Read the model definition and answer for the solid it produces. Units are mm, in the model's axes. Coordinates: 2 decimals unless noted, no trailing zeros. Loops run counter-clockwise (first coordinate to the right, second up) from the corner with the lowest first, then second, coordinate; pieces in that order, holes last. Notation, with made-up numbers: M -29,37 L 10,37 A8 cw 10,50 Z; hole C 6.5,46.5 d11. An arc over 180 degrees is marked long. Put each result on its own line as item: value.
from build123d import *

# Parameters (mm, degrees)
BOSS_EXTRUDE2_REACH      = 243.079
BOSS_EXTRUDE2_END_RADIUS = 266.319
SKETCH10_R               = 25.4
SKETCH11_R               = 12.7
CUT_EXTRUDE1_DEPTH       = 190.754
CIRPATTERN1_COUNT        = 6


with BuildPart() as part:
    # Sketch1 → Revolve1 (revolve)
    with BuildSketch(Plane(origin=(0, 0, 0), x_dir=(1, 0, 0), z_dir=(0, 1, 0)), mode=Mode.PRIVATE) as revolve1_sk:
        with BuildLine():
            Line((-148.59, 0), (-140.97, 0))
            Line((-140.97, 0), (-140.97, 12.391039743))
            ThreePointArc((-140.97, 12.391039743), (-134.615921102, 34.866271953), (-117.434796957, 50.687755913))
            ThreePointArc((-117.434796957, 50.687755913), (-60.367509579, 71.617582047), (0, 78.72368491))
            Line((0, 78.72368491), (0, 85.07368491))
            ThreePointArc((0, 85.07368491), (-61.842045719, 77.794008454), (-120.303258046, 56.352950612))
            ThreePointArc((-120.303258046, 56.352950612), (-131.462846302, 48.602983737), (-140.081763243, 38.1))
            Line((-140.081763243, 38.1), (-149.225, 38.1))
            Line((-149.225, 38.1), (-149.225, 25.4))
            Line((-149.225, 25.4), (-152.4, 25.4))
            Line((-152.4, 25.4), (-156.21, 13.674025723))
            Line((-156.21, 13.674025723), (-156.21, 9.503030405))
            Line((-156.21, 9.503030405), (-152.4, 12.7))
            Line((-152.4, 12.7), (-148.59, 12.7))
            Line((-148.59, 12.7), (-148.59, 0))
        make_face()
    revolve(revolve1_sk.sketch.rotate(Axis((0, 0, -78.72368491), (0, 0, -1)), 180), axis=Axis((0, 0, -78.72368491), (0, 0, -1)))

    # Boss-Extrude2: up to this sphere (the profile starts outside it)
    boss_extrude2_end = Location((0, 0, 181.24531509)) * Sphere(BOSS_EXTRUDE2_END_RADIUS, mode=Mode.PRIVATE)
    # Sketch10 → Boss-Extrude2 (add, up to the surface)
    with BuildSketch(Plane.XY.offset(-96.52), mode=Mode.PRIVATE) as boss_extrude2_sk1:
        Circle(SKETCH10_R)
    boss_extrude2_tool1 = extrude(boss_extrude2_sk1.sketch, amount=BOSS_EXTRUDE2_REACH, mode=Mode.PRIVATE) - boss_extrude2_end
    add(boss_extrude2_tool1.solids().sort_by_distance((0, 0, -96.52))[0])

    # Sketch11 → Cut-Extrude1 (cut)
    with BuildSketch(Plane.XY):
        Circle(SKETCH11_R)
    extrude(amount=-CUT_EXTRUDE1_DEPTH, mode=Mode.SUBTRACT)

    # Sketch15 → 1/4 (0.25) Diameter Hole1 (revolve, cut)
    with BuildSketch(Plane(origin=(149.225, 0, -31.75), x_dir=(0, 0, -1), z_dir=(0, 1, 0))):
        Polygon((0, 0), (0, 8.257732465), (3.175, 6.35), (3.175, 0), align=None)
    f_1_4_0_25_diameter_hole1 = revolve(axis=Axis((155.575, 0, -31.75), (-1, 0, 0)), mode=Mode.SUBTRACT)

    # CirPattern1: 1/4 (0.25) Diameter Hole1 ×6 about axis
    cirpattern1_axis = Axis((0, 0, 5.473137056), (0, 0, -1))
    for i in range(1, CIRPATTERN1_COUNT):
        add(f_1_4_0_25_diameter_hole1.rotate(cirpattern1_axis, i * 360 / CIRPATTERN1_COUNT), mode=Mode.SUBTRACT)

    # Fillet1: read off the stored shape, not the designer's step
    # Fillet1 outline → Fillet1 (revolve, cut)
    with BuildSketch(Plane.XZ):
        with BuildLine():
            ThreePointArc((12.7, -80.82093127), (13.39254924, -79.077794531), (15.092539913, -78.285215291))
            Line((15.092539913, -78.285215291), (12.7, -78.285215291))
            Line((12.7, -78.285215291), (12.7, -80.82093127))
        make_face()
    revolve(axis=Axis((0, 0, 0), (0, 0, 1)), mode=Mode.SUBTRACT)


solid = part.part
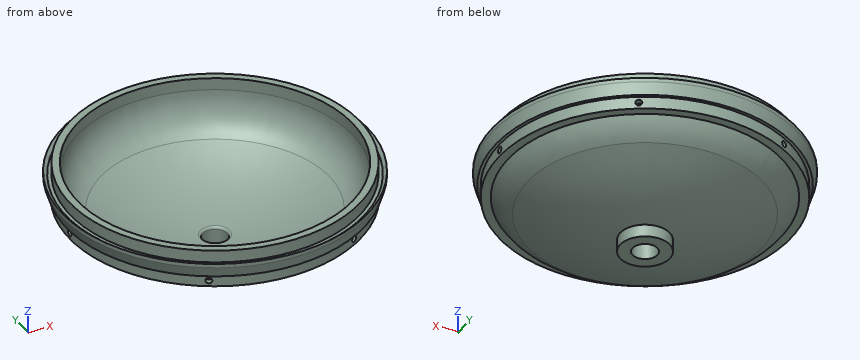
1) Given pin 1 Ø5 at (x, y) = (-51, -68) entering from -Z; pin 2 Ø10 at (x, z) = (-116.5, -17) entering from +Y; pin 3 Ø10 at (y, z) = (0, -31.75) entering from -X (3 decimals), each flat-ended and moving along its own axis, determine where each tip first touches the part or whether it passes through.
Answer list:
pin 1: stops at z = -71.97
pin 2: stops at y = 108.36
pin 3: stops at x = -149.225
2) Straight lines are drawn through the part: line 1 (Y direction, x = 0, z = -8); line 2 (Y direction, x = 100.5, z = -44); line 3 (X direction, y = 7.5, z = -52.5). For each, find the intervals that lie inside material, in ascending order. Write a range as [from, to].
Answer list:
line 1: y = [-148.59, -140.97], [140.97, 148.59]
line 2: y = [-91.4, -77.79], [77.79, 91.4]
line 3: x = [-126.45, -113.54], [113.54, 126.45]
3) Find section B-B, the plane z = -43. Write down the section's boundary in (x, y).
Answer list:
outline: C 0,0 d273.32; hole C 0,0 d256.28
4) Find section A-A, the plane z = -87.5. Write down the section's boundary in (x, y), plus the area to 3 significant figures.
Answer list:
outline: C 0,0 d50.8; hole C 0,0 d25.4
area: 1,520 mm^2
